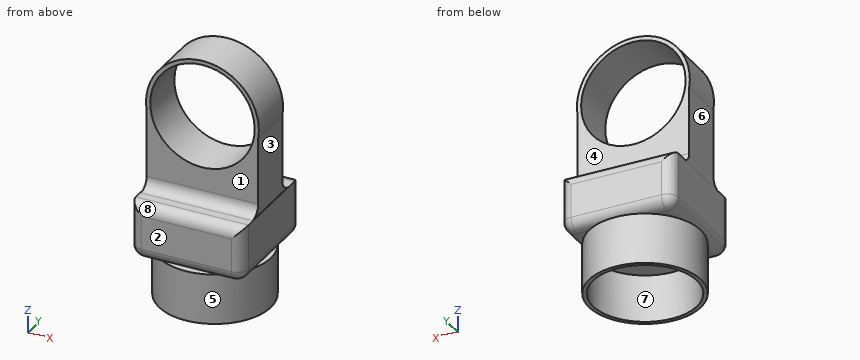
```python
from build123d import *

# Parameters (mm, degrees)
SKETCH_1_R          = 50.5
SKETCH_1_R_2        = 46.75
EXTRUDE_1_DEPTH     = 42.3
EXTRUDE_3_DEPTH     = 42.3
SKETCH_10_W         = 100.829972986
SKETCH_10_H         = 100
EXTRUDE_6_DEPTH     = 50
FILLET_13_R         = 10
FILLET_14_R         = 10
SKETCH_11_R         = 50
EXTRUDE_7_DEPTH     = 45
SKETCH_12_R         = 46.5
CUT_EXTRUDE_1_DEPTH = 42.3


with BuildPart() as part:
    # 草图1 → 凸台-拉伸1 (new body)
    with BuildSketch(Plane(origin=(0, 0, 0), x_dir=(1, 0, 0), z_dir=(0, 1, 0))):
        with Locations(Location((0, 0, 0), (0, 0, 270))):
            Circle(SKETCH_1_R)
        with Locations(Location((0, 0, 0), (0, 0, 270))):
            Circle(SKETCH_1_R_2, mode=Mode.SUBTRACT)
    extrude(amount=EXTRUDE_1_DEPTH)

    # 草图2 → 凸台-拉伸3 (add)
    with BuildSketch(Plane(origin=(0, 42.3, 0), x_dir=(1, 0, 0), z_dir=(0, 1, 0))):
        with BuildLine():
            Line((-49.922748528, 77.584165112), (49.927251472, 77.584165112))
            Line((49.927251472, 77.584165112), (49.927251472, 7.584165112))
            ThreePointArc((49.927251472, 7.584165112), (0.002251472, 49.671200662), (-49.922748528, 7.584165112))
            Line((-49.922748528, 7.584165112), (-49.922748528, 77.584165112))
        make_face()
    extrude(amount=-EXTRUDE_3_DEPTH)

    # 草图10 → 凸台-拉伸6 (add)
    with BuildSketch(Plane(origin=(0, 0, -77.584165112), x_dir=(-1, 0, 0), z_dir=(0, 0, -1))):
        with Locations((0, 21.964414078)):
            Rectangle(SKETCH_10_W, SKETCH_10_H)
    extrude(amount=EXTRUDE_6_DEPTH)

    # 圆角13
    fillet_13_edges = [part.edges().sort_by_distance(p)[0] for p in [
        (0.002251472, 0, -77.584165112),
        (0.002251472, 42.3, -77.584165112),
    ]]
    fillet(fillet_13_edges, radius=FILLET_13_R)

    # 圆角14
    fillet_14_edges = [part.edges().sort_by_distance(p)[0] for p in [
        (-50.414986493, -28.035585922, -102.584165112),
        (0, 71.964414078, -77.584165112),
        (-50.414986493, 71.964414078, -102.584165112),
        (50.414986493, 71.964414078, -102.584165112),
        (0, -28.035585922, -77.584165112),
        (50.414986493, -28.035585922, -102.584165112),
        (-50.414986493, 21.964414078, -127.584165112),
        (0, 71.964414078, -127.584165112),
        (50.414986493, 21.964414078, -127.584165112),
        (0, -28.035585922, -127.584165112),
    ]]
    fillet(fillet_14_edges, radius=FILLET_14_R)

    # 草图11 → 凸台-拉伸7 (add)
    with BuildSketch(Plane(origin=(0, 0, -127.584165112), x_dir=(-1, 0, 0), z_dir=(0, 0, -1))):
        with Locations(Location((0, 21.964414078, 0), (0, 0, 143.930141518))):
            Circle(SKETCH_11_R)
    extrude(amount=EXTRUDE_7_DEPTH)

    # 草图12 → 切除-拉伸1 (cut)
    with BuildSketch(Plane(origin=(0, 0, -172.584165112), x_dir=(-1, 0, 0), z_dir=(0, 0, -1))):
        with Locations((0, 21.964414078)):
            Circle(SKETCH_12_R)
    extrude(amount=-CUT_EXTRUDE_1_DEPTH, mode=Mode.SUBTRACT)


solid = part.part
```
Model file for the job. Use its own axes, mm. Face numbers are marked on the shaded views. A direction names the side the tool comes from. Round coordinates to 2 decimals unless told otherwise and drop trailing zeros. Write each loop counter-clockwise with the first axis right and the second up, starting at its lowest first coordinate (ties: lowest second). Pieces come first, ordered by that corner, then holes. Notation, with made-up numbers: (8, 4) - (49, 4) arc R35 cw to (49, 38) - close; hole circle Ø1 at (-11.5, -34). An arc over 180 degrees is marked (long way). One line per item, written item: value.
(1) Cut at C-C, the plane y = 4. Give the cut face in (x, z).
Values follow:
outline: (-50.41, -117.58) arc R10 ccw to (-40.41, -127.58) - (-46.66, -127.58) - (-46.66, -172.58) - (-42.89, -172.58) - (-42.89, -130.28) - (42.89, -130.28) - (42.89, -172.58) - (46.66, -172.58) - (46.66, -127.58) - (40.41, -127.58) arc R10 ccw to (50.41, -117.58) - (50.41, -77.58) - (49.93, -77.58) - (49.93, -7.58) arc R50.5 ccw (long way) to (-49.92, -7.61) - (-49.92, -77.58) - (-50.41, -77.58) - close; hole circle Ø93.5 at (0, 0)
(2) 3-axis set-ups, long thin cutter, end or side, ignore diameter. For the marked faces 1, 2, 3, 4 and 5: which of +Z, -Z, +X, -X, +Y, -Y reach the whole face in a straight line?
Values follow:
face 1: +Z, +X, -X, -Y
face 2: +Z, -Z, +X, -X, -Y
face 3: +X, +Y, -Y
face 4: +Z, +X, -X, +Y
face 5: -Z
(3) Cut at B-B, the plane z = 0. Give the cut face in (x, y), plus the area to 3 significant figures.
Values follow:
outline: (-50.5, 0) - (-46.75, 0) - (-46.75, 42.3) - (-50.5, 42.3) - close; (46.75, 0) - (50.5, 0) - (50.5, 42.3) - (46.75, 42.3) - close
area: 317 mm²
(4) Two-plate mould, pull along Z, no slides. Class the marked faces 6, 7 and 8: pulls with the +Z half, pulls with the -Z half, needs draft (parallel to the pull), parting line crosses it, or undercut.
Values follow:
face 6: undercut
face 7: needs draft
face 8: pulls with the +Z half
(5) Wall check: probe 1 along Y at (x, z) = (0, -150); probe 2 along Z at (x, y) = (-43, 14); probe 3 along X at (y, z) = (24, 0). Give the ranges that are in metal, low to high.
Values follow:
probe 1: y = -28.04 to -24.54, 68.46 to 71.96
probe 2: z = -130.28 to -127.58, -127.24 to -18.35, 18.35 to 26.48
probe 3: x = -50.5 to -46.75, 46.75 to 50.5
(6) Cut at D-D, the plane x = 17. Give the cut face in (y, z).
Values follow:
outline: (-28.04, -117.58) arc R10 ccw to (-18.04, -127.58) - (-25.06, -127.58) - (-25.06, -172.58) - (-21.32, -172.58) - (-21.32, -130.28) - (65.25, -130.28) - (65.25, -172.58) - (68.99, -172.58) - (68.99, -127.58) - (61.96, -127.58) arc R10 ccw to (71.96, -117.58) - (71.96, -87.58) arc R10 ccw to (61.96, -77.58) - (52.3, -77.58) arc R10 cw to (42.3, -67.58) - (42.3, -43.55) - (0, -43.55) - (0, -67.58) arc R10 cw to (-10, -77.58) - (-18.04, -77.58) arc R10 ccw to (-28.04, -87.58) - close; (0, 43.55) - (42.3, 43.55) - (42.3, 47.55) - (0, 47.55) - close
(7) Cut at A-A, the plane x = 0. Give the cut face in (y, z), plus the area to 3 significant figures.
Values follow:
outline: (-28.04, -172.58) - (-24.54, -172.58) - (-24.54, -130.28) - (68.46, -130.28) - (68.46, -172.58) - (71.96, -172.58) - (71.96, -127.58) - (61.96, -127.58) arc R10 ccw to (71.96, -117.58) - (71.96, -87.58) arc R10 ccw to (61.96, -77.58) - (52.3, -77.58) arc R10 cw to (42.3, -67.58) - (42.3, -46.75) - (0, -46.75) - (0, -67.58) arc R10 cw to (-10, -77.58) - (-18.04, -77.58) arc R10 ccw to (-28.04, -87.58) - (-28.04, -117.58) arc R10 ccw to (-18.04, -127.58) - (-28.04, -127.58) - close; (0, 46.75) - (42.3, 46.75) - (42.3, 50.5) - (0, 50.5) - close
area: 6,990 mm²
(8) Drop flat-ended pins along their axis: P1, Ø8, axis at y = 58, z = -106.5, coming from the -X side (3 decimals); P2, Ø6, axis at x = -17.5, y = 43.5, coming from the -Z side; P3, Ø11, axis at x = 1, y = 68, coming from the +Z side. Give the stop position or say it passes through.
Values follow:
P1: stops at x = -50.415
P2: stops at z = -130.28
P3: stops at z = -77.6
